For this review, take the finished solid that the model builds, in its own axes (mm). A direction names the side the tool comes from. Give positions to 0.01 mm unless a question says otherwise; leave off trailing zeros. Order: outer loops, then holes, each group sorted by start corner. A loop starts at its lowest first (then second) coordinate and runs counter-clockwise, first axis right, second up.
from build123d import *

# Parameters (mm, degrees)
F0_W     = 370
F0_H     = 320
F1_DEPTH = 70
F2_W     = 332
F2_H     = 282
F3_DEPTH = 51
F4_W     = 348
F4_H     = 140
F4_W_2   = 320
F4_H_2   = 70
F5_DEPTH = 19
F6_W     = 80
F6_H     = 20
F7_DEPTH = 19


with BuildPart() as f1:
    # F0 (on Top) → F1 (new body)
    with BuildSketch(Plane.XY):
        Rectangle(F0_W, F0_H)
    extrude(amount=F1_DEPTH)

    # F2 (on face) → F3 (cut)
    with BuildSketch(Plane.XY.offset(70)):
        Rectangle(F2_W, F2_H)
    extrude(amount=-F3_DEPTH, mode=Mode.SUBTRACT)

    # F4 (on face) → F5 (join)
    with BuildSketch(Plane.YZ.offset(185)):
        with Locations((0, 35)):
            Rectangle(F4_W, F4_H)
        with Locations((0, 35)):
            Rectangle(F4_W_2, F4_H_2, mode=Mode.SUBTRACT)
        with Locations((0, 35)):
            Rectangle(F4_W_2, F4_H_2)
    extrude(amount=F5_DEPTH)

    # F6 (on face) → F7 (join)
    with BuildSketch(Plane.YZ.offset(204)):
        with Locations((0, 35)):
            Rectangle(F6_W, F6_H)
    extrude(amount=F7_DEPTH)


solid = f1.part
1) Tool access review of faces 5 (the face through (-3, 2, 0)), 6 (the face through (-3, -160, 35)), 7 (the face through (-14.6, -141.5, 70)), 8 (the face through (-166, -2, 45)), 9 (the face through (213, -1, 45)): name each direction out of +Z, -Z, +X, -X, +Y, -Y from which nothing blocks a thin tool from reaching the whole face with its end or side.
Answer sheet:
face 5: -Z, -X, +Y, -Y
face 6: +Z, -Z, -X, -Y
face 7: +Z, -X, +Y, -Y
face 8: +Z
face 9: +Z, +X, +Y, -Y
2) Clearance check with flat-ended pins moving along their axes: pin 1 (12 mm diameter, centred on y = 135, z = 44, fed in from +X); pin 2 (9.5 mm diameter, centred on x = 214, y = -7.5, fed in from -Z); pin 3 (3 mm diameter, centred on x = 126, y = 2, fed in from +Z); pin 4 (12 mm diameter, centred on x = 68, z = 78, fed in from +Y). State where each tip first meets the part, or that it passes through.
Answer sheet:
pin 1: stops at x = 204
pin 2: stops at z = 25
pin 3: stops at z = 19
pin 4: passes through
3) We need section C-C on x = -151. Give the boundary of the cut face in (y, z).
Answer sheet:
outline: (-160, 0) - (160, 0) - (160, 70) - (141, 70) - (141, 19) - (-141, 19) - (-141, 70) - (-160, 70) - close
4) We need section D-D on z = 6. Give the boundary of the cut face in (x, y).
Answer sheet:
outline: (-185, -160) - (185, -160) - (185, -174) - (204, -174) - (204, 174) - (185, 174) - (185, 160) - (-185, 160) - close
5) To check wall thickness, follow line 1 (X direction, y = 7, z = 19.5); line 2 (Z direction, x = 10, y = -97); line 3 (X direction, y = 25.5, z = 42.5). State the ranges of each line that lie inside material, in increasing order.
Answer sheet:
line 1: x = -185 to -166, 166 to 204
line 2: z = 0 to 19
line 3: x = -185 to -166, 166 to 223
6) We need section B-B on y = -64.5. Give the boundary of the cut face in (x, z), then the cut area to 3 significant figures.
Answer sheet:
outline: (-185, 0) - (185, 0) - (185, -35) - (204, -35) - (204, 105) - (185, 105) - (185, 70) - (166, 70) - (166, 19) - (-166, 19) - (-166, 70) - (-185, 70) - close
area: 11,600 mm2
7) Draft analysis for pull direction Y (two halves, no side actions). For faces 1 (the face through (-2, 141, 45)), 2 (the face through (-2, 2, 19)), 3 (the face through (194, -2, -35)), 4 (the face through (213, -40, 35)), state which applies: +Y half, -Y half, draft (parallel to the pull), parting line (faces both ways), or undercut.
Answer sheet:
face 1: undercut
face 2: undercut
face 3: draft
face 4: -Y half
8) We need section A-A on z = 59.5. Give the boundary of the cut face in (x, y), then the cut area to 3 significant figures.
Answer sheet:
outline: (-185, -160) - (185, -160) - (185, -174) - (204, -174) - (204, 174) - (185, 174) - (185, 160) - (-185, 160) - close; hole (-166, -141) - (166, -141) - (166, 141) - (-166, 141) - close
area: 31,400 mm2
